Design review of the part built by this model. Coordinates are the model's own, in mm. Face numbers are marked on the shaded views. A direction names the side the tool comes from. Give positions to 0.01 mm unless a question says otherwise; leave off trailing zeros. Write each loop counter-clockwise with the first axis right and the second up, starting at its lowest first coordinate (ties: lowest second). Pieces come first, ordered by that corner, then holes. Notation, with made-up numbers: (-18.75, -26) -> (-13.75, -26) arc R17 ccw to (-13.75, -11) -> close; hole circle Ø9 at (35.25, 42). An arc over 180 degrees is marked (long way). Use CSV: the item, a comma, the result in double quotes.
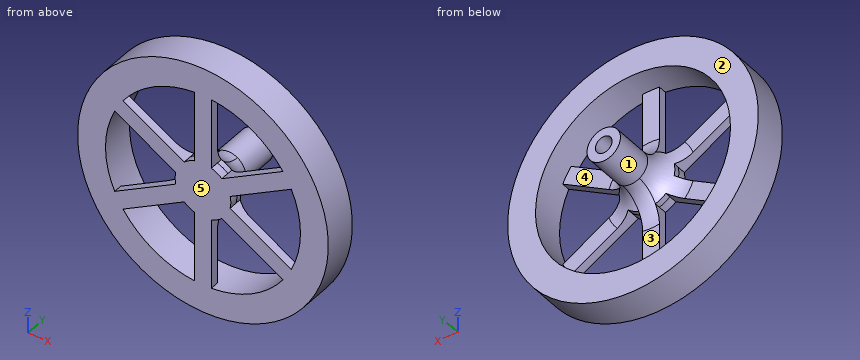
```python
from build123d import *

# Parameters (mm, degrees)
SKETCH2_R           = 45
SKETCH2_R_2         = 35
BOSS_EXTRUDE1_DEPTH = 12
BOSS_EXTRUDE2_DEPTH = 3
CIRPATTERN1_COUNT   = 6
SKETCH4_R           = 6
SKETCH4_R_2         = 3
BOSS_EXTRUDE3_DEPTH = 23.6
FILLET1_R           = 10


with BuildPart() as part:
    # Sketch2 → Boss-Extrude1 (new body)
    with BuildSketch(Plane(origin=(0, 0, 0), x_dir=(1, 0, 0), z_dir=(0, 1, 0))):
        with Locations(Location((0, 0, 0), (0, 0, 270))):
            Circle(SKETCH2_R)
        with Locations(Location((0, 0, 0), (0, 0, 270))):
            Circle(SKETCH2_R_2, mode=Mode.SUBTRACT)
    extrude(amount=BOSS_EXTRUDE1_DEPTH)

    # Sketch3 → Boss-Extrude2 (add)
    with BuildSketch(Plane.XZ):
        with BuildLine():
            Line((-3, 40.114762923), (3, 40.114762923))
            Line((3, 40.114762923), (3, 9.539392014))
            ThreePointArc((3, 9.539392014), (0, -10), (-3, 9.539392014))
            Line((-3, 9.539392014), (-3, 40.114762923))
        make_face()
    boss_extrude2 = extrude(amount=-BOSS_EXTRUDE2_DEPTH)

    # CirPattern1: Boss-Extrude2 ×6 about axis
    cirpattern1_axis = Axis((0, 0, 0), (0, 1, 0))
    for i in range(1, CIRPATTERN1_COUNT):
        add(boss_extrude2.rotate(cirpattern1_axis, i * 360 / CIRPATTERN1_COUNT))

    # Sketch4 → Boss-Extrude3 (add)
    with BuildSketch(Plane(origin=(0, 3, 0), x_dir=(1, 0, 0), z_dir=(0, 1, 0))):
        with Locations(Location((0, 0, 0), (0, 0, 90))):
            Circle(SKETCH4_R)
        with Locations(Location((0, 0, 0), (0, 0, 270))):
            Circle(SKETCH4_R_2, mode=Mode.SUBTRACT)
    extrude(amount=BOSS_EXTRUDE3_DEPTH)

    # Fillet1
    # the kernel refuses this fillet: 10 mm, written as the material it adds along each edge
    with BuildSketch(Plane(origin=(0, 3, 0), x_dir=(0, 0, -1), z_dir=(1, 0, 0))) as fillet1_piece_1_section:
        with BuildLine():
            CenterArc((6 + FILLET1_R, FILLET1_R), FILLET1_R, 180, 90)
            Line((6, FILLET1_R), (6, 0))
            Line((6, 0), (6 + FILLET1_R, 0))
        make_face()
    fillet1_piece_1 = revolve(axis=Axis((0, 3, 0), (0, 1, 0)), mode=Mode.PRIVATE)
    fillet1_piece_1 = split(fillet1_piece_1, bisect_by=Plane(origin=(3, 3.588688927, -11.330954683), z_dir=(-1, 0, 0)), keep=Keep.TOP, mode=Mode.PRIVATE)
    fillet1_piece_1 = split(fillet1_piece_1, bisect_by=Plane(origin=(-3, 3.588688927, -11.330954683), z_dir=(1, 0, 0)), keep=Keep.TOP, mode=Mode.PRIVATE)
    add(fillet1_piece_1)
    with BuildSketch(Plane(origin=(0, 3, 0), x_dir=(0, 0, -1), z_dir=(1, 0, 0))) as fillet1_piece_2_section:
        with BuildLine():
            CenterArc((6 + FILLET1_R, FILLET1_R), FILLET1_R, 180, 90)
            Line((6, FILLET1_R), (6, 0))
            Line((6, 0), (6 + FILLET1_R, 0))
        make_face()
    fillet1_piece_2 = revolve(axis=Axis((0, 3, 0), (0, 1, 0)), mode=Mode.PRIVATE)
    fillet1_piece_2 = fillet1_piece_2 & Plane(origin=(0, 4.321014417, 0), x_dir=(0.2999999999999998, 0, 0.9539392014169458), z_dir=(0, -1, 0)) * Cylinder(10, 64, mode=Mode.PRIVATE)
    add(fillet1_piece_2)
    with BuildSketch(Plane(origin=(0, 3, 0), x_dir=(0, 0, -1), z_dir=(1, 0, 0))) as fillet1_piece_3_section:
        with BuildLine():
            CenterArc((6 + FILLET1_R, FILLET1_R), FILLET1_R, 180, 90)
            Line((6, FILLET1_R), (6, 0))
            Line((6, 0), (6 + FILLET1_R, 0))
        make_face()
    fillet1_piece_3 = revolve(axis=Axis((0, 3, 0), (0, 1, 0)), mode=Mode.PRIVATE)
    fillet1_piece_3 = split(fillet1_piece_3, bisect_by=Plane(origin=(-11.312894604, 3.588688928, -3.06740113), z_dir=(0.5000000000000002, 0, -0.8660254037844386)), keep=Keep.TOP, mode=Mode.PRIVATE)
    fillet1_piece_3 = split(fillet1_piece_3, bisect_by=Plane(origin=(-8.312894604, 3.588688928, -8.263553553), z_dir=(-0.5000000000000001, 0, 0.8660254037844387)), keep=Keep.TOP, mode=Mode.PRIVATE)
    add(fillet1_piece_3)
    with BuildSketch(Plane(origin=(0, 3, 0), x_dir=(0, 0, -1), z_dir=(1, 0, 0))) as fillet1_piece_4_section:
        with BuildLine():
            CenterArc((6 + FILLET1_R, FILLET1_R), FILLET1_R, 180, 90)
            Line((6, FILLET1_R), (6, 0))
            Line((6, 0), (6 + FILLET1_R, 0))
        make_face()
    fillet1_piece_4 = revolve(axis=Axis((0, 3, 0), (0, 1, 0)), mode=Mode.PRIVATE)
    fillet1_piece_4 = split(fillet1_piece_4, bisect_by=Plane(origin=(11.312894604, 3.588688928, -3.06740113), z_dir=(-0.4999999999999998, 0, -0.8660254037844388)), keep=Keep.TOP, mode=Mode.PRIVATE)
    fillet1_piece_4 = split(fillet1_piece_4, bisect_by=Plane(origin=(8.312894604, 3.588688928, -8.263553553), z_dir=(0.49999999999999994, 0, 0.8660254037844389)), keep=Keep.TOP, mode=Mode.PRIVATE)
    add(fillet1_piece_4)


solid = part.part
```
(1) Tool access review of the marked faces 4 and 5: name each direction out of +Z, -Z, +X, -X, +Y, -Y from which nothing blocks a thin tool from reaching the whole face with its end or side.
Established:
face 4,"+Y"
face 5,"+Z, -Z, +X, -X, -Y"
(2) Take a section at D-D (y = 22). Write out the cut boundary in (x, z).
Established:
outline,"circle Ø12 at (0, 0); hole circle Ø6 at (0, 0)"
(3) For line 1 along X through (y, z) = (21, 0); line 2 along X through (y, z) = (11.5, 0); line 3 along Z through (x, y) = (4, 8.5), list the stretches that pass through material, from the lowest coordinate up. Write a range as [from, to].
Established:
line 1,"x = [-6, -3], [3, 6]"
line 2,"x = [-45, -35], [-6.11, -3], [3, 6.11], [35, 45]"
line 3,"z = [-44.82, -34.77], [-5.83, 5.83], [34.77, 44.82]"
(4) Mouldability with a two-part tool opening along X and no side actions: class the marked faces 1, 2 and 3 as +X half, -X half, draft (parallel to the pull), parting line (faces both ways), or undercut.
Established:
face 1,"parting line"
face 2,"draft"
face 3,"undercut"
(5) Clearance check with flat-ended pins moving along their axes: pin 1 (12 mm diameter, centred on x = -18, z = 12.5, fed in from +Y); pin 2 (1 mm diameter, centred on y = 21.5, z = 1, fed in from +X); pin 3 (6 mm diameter, centred on x = 10.5, z = 14, fed in from -Y); pin 4 (1 mm diameter, centred on x = -20.5, y = 11.5, fed in from +Z). State where each tip first meets the part, or that it passes through.
Established:
pin 1,"stops at y = 3"
pin 2,"stops at x = 5.98"
pin 3,"passes through"
pin 4,"stops at z = 40.31"
(6) Take a section at A-A (z = 0). Write out the cut boundary in (x, y).
Established:
outline,"(-45, 0) -> (-35, 0) -> (-35, 12) -> (-45, 12) -> close; (-10, 0) -> (10, 0) -> (10, 5) arc R10 cw to (6, 13) -> (6, 26.6) -> (3, 26.6) -> (3, 3) -> (-3, 3) -> (-3, 26.6) -> (-6, 26.6) -> (-6, 13) arc R10 cw to (-10, 5) -> close; (35, 0) -> (45, 0) -> (45, 12) -> (35, 12) -> close"
(7) Take a section at C-C (x = -21.5). Write out the cut boundary in (y, z), then the cut area to 3 significant figures.
Established:
outline,"(0, -39.53) -> (12, -39.53) -> (12, -27.62) -> (0, -27.62) -> close; (0, -15.88) -> (3, -15.88) -> (3, -8.95) -> (0, -8.95) -> close; (0, 8.95) -> (3, 8.95) -> (3, 15.88) -> (0, 15.88) -> close; (0, 27.62) -> (12, 27.62) -> (12, 39.53) -> (0, 39.53) -> close"
area,"327 mm2"
(8) Take a section at B-B (x = 0). Write out the cut boundary in (y, z).
Established:
outline,"(0, -45) -> (12, -45) -> (12, -35) -> (3, -35) -> (3, -16) arc R10 cw to (13, -6) -> (26.6, -6) -> (26.6, -3) -> (3, -3) -> (3, 3) -> (26.6, 3) -> (26.6, 6) -> (13, 6) arc R10 cw to (3, 16) -> (3, 35) -> (12, 35) -> (12, 45) -> (0, 45) -> close"
